Could you check a few things on this model? Use its own coordinates, in mm. Face numbers are marked on the shaded views. A direction names the side the tool comes from. Coordinates: 2 decimals unless noted, no trailing zeros. Loops run counter-clockwise (first coordinate to the right, second up) from the corner with the lowest first, then second, coordinate; pieces in that order, holes last. Notation, with made-up numbers: (42.5, 46) - (72.5, 46) arc R9 cw to (72.5, 52) - close; hole circle Ø3 at (67.5, 71). An arc over 180 degrees is marked (long way). One line per item, written item: value. Start each with the question number.
(1) If I drill on line 1 along X through (y, z) = (0, -6.15); line 2 along Y through (x, z) = (8.5, 0); line 3 along Y through (x, z) = (3.5, 5.65), over which ranges is the centre line in solid material (lowest first)? Write a range as from..to.
(2) If we section it at C-C on y = 0: Count the separate pieces of the cut face and the enclosed holes in it, then the cut area to 4 significant figures.
(3) If we section it at D-D on x = 14: Write out the boundary of the cut face in (y, z), then the cut area to 3 significant figures.
(4) If we section it at B-B on x = 3.5: Write out the boundary of the cut face in (y, z).
(5) I'm going to push flat-ended pins straight in: P1, Ø4, axis at x = 3.5, y = 0, coming from the -Z side; P2, Ø5, axis at x = 16.5, y = 6, coming from the -Z side; P3, Ø3, axis at x = 15.5, z = -8.5, coming from the -Y side. Where does each tip first touch, or does it pass through?
(6) If we mould it in two halves opening along Z, with no side actions, what happens to the marked faces 5, 6 and 7? For each: pulls with the +Z half, pulls with the -Z half, needs draft (parallel to the pull), parting line crosses it, or undercut.
(7) On a 3-axis mill with a long thin cutter (end or side, diameter ignored), from which of +Z, -Z, +X, -X, +Y, -Y can I reach the whole of each face in a straight line? I mean the marked faces 1, 2, 3 and 4. Say none if no direction works.
```python
from build123d import *

# Parameters (mm, degrees)
SKETCH2_R          = 4
CUT_EXTRUDE1_DEPTH = 29.222331583
SKETCH3_R          = 1.5
CUT_EXTRUDE2_DEPTH = 20
FILLET1_R          = 0.5


with BuildPart() as part:
    # Sketch1 → Revolve1 (revolve)
    with BuildSketch(Plane.XY, mode=Mode.PRIVATE) as revolve1_sk:
        Polygon((0, 0), (0, 7.5), (8, 7.5), (8, 12.5), (9.5, 12.5), (13, 9), (16.5, 12.5), (18, 12.5), (18, 7.5), (22, 7.5), (22, 0), align=None)
    revolve(revolve1_sk.sketch.rotate(Axis((22, 0, 0), (-1, 0, 0)), 90), axis=Axis((22, 0, 0), (-1, 0, 0)))

    # Sketch2 → Cut-Extrude1 (cut, through all)
    with BuildSketch(Plane(origin=(22, 0, 0), x_dir=(0, 0, -1), z_dir=(1, 0, 0))):
        Circle(SKETCH2_R)
    extrude(amount=-CUT_EXTRUDE1_DEPTH, mode=Mode.SUBTRACT)

    # Sketch3 → Cut-Extrude2 (cut, symmetric)
    with BuildSketch(Plane.XY):
        with Locations((3.5, 0)):
            Circle(SKETCH3_R)
    extrude(amount=CUT_EXTRUDE2_DEPTH, both=True, mode=Mode.SUBTRACT)

    # Fillet1
    fillet1_edges = [part.edges().sort_by_distance(p)[0] for p in [
        (8, 0, 7.5),
        (0, 0, 7.5),
        (22, 0, 7.5),
        (18, 0, 7.5),
    ]]
    fillet(fillet1_edges, radius=FILLET1_R)


solid = part.part
```
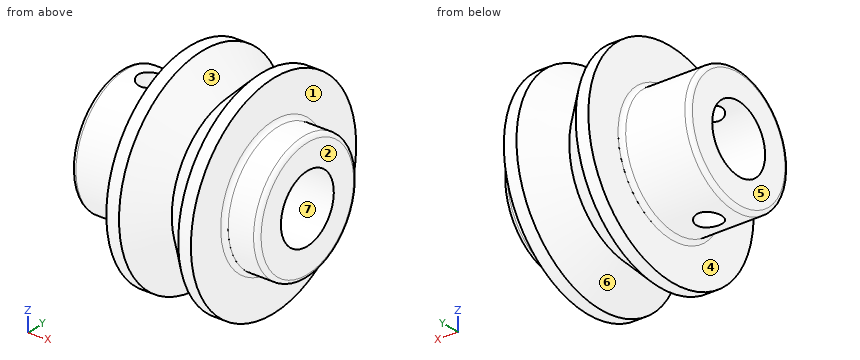
Values:
1. line 1: x = 0..2, 5..22
1. line 2: y = -12.5..-4, 4..12.5
1. line 3: y = -4.93..-1.5, 1.5..4.93
2. separate pieces: 4
2. enclosed holes: 0
2. area: 208.5 mm2
3. outline: circle Ø20 at (0, 0); hole circle Ø8 at (0, 0)
3. area: 264 mm2
4. outline: (-1.5, -7.35) - (-1.5, -3.71) arc R4 cw to (-1.5, 3.71) - (-1.5, 7.35) arc R7.5 ccw to start; (1.5, -7.35) arc R7.5 ccw to (1.5, 7.35) - (1.5, 3.71) arc R4 cw to (1.5, -3.71) - close
5. P1: stops at z = -7.5
5. P2: stops at z = -12
5. P3: stops at y = -10.09
6. face 5: needs draft
6. face 6: parting line crosses it
6. face 7: undercut
7. face 1: +X
7. face 2: +Z, -Z, +X, +Y, -Y
7. face 3: none
7. face 4: -X
